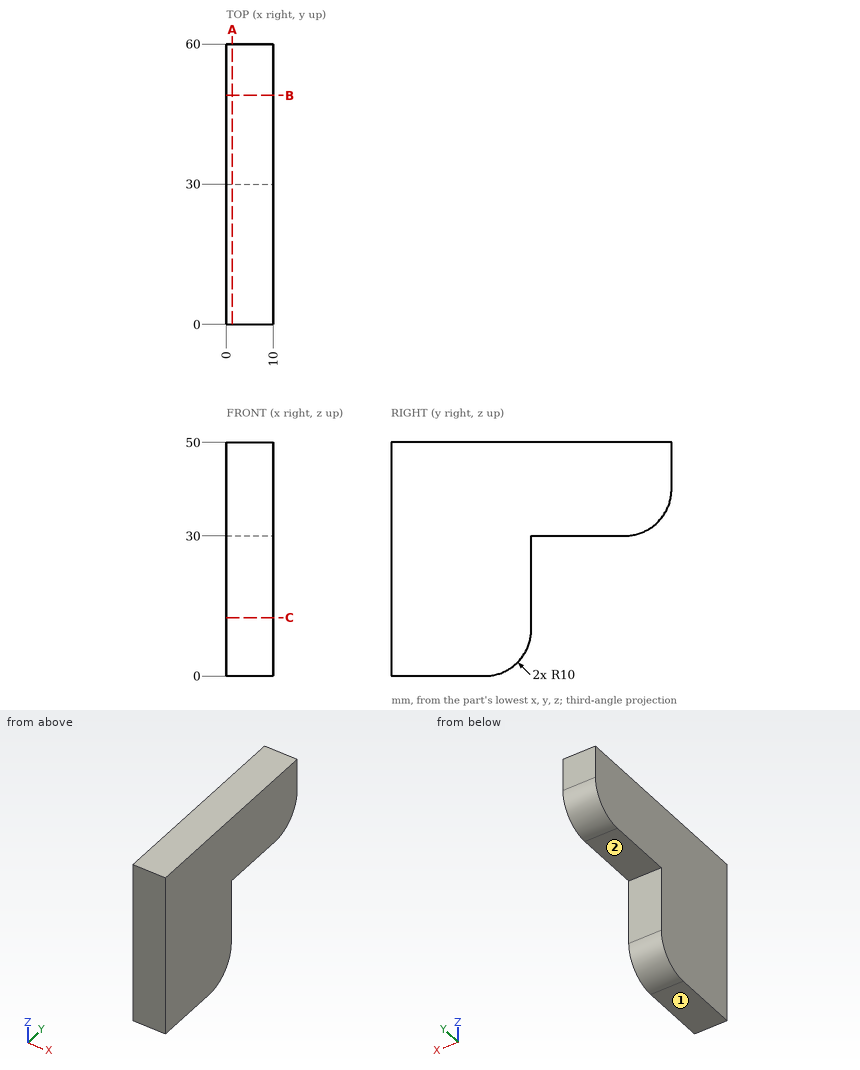
The figure shows three views and two pictorial views of one solid part (mm, origin at its lowest corner). Answer the questions. A direction names the side the tool comes from. Give positions to 0.01 mm unless a question says otherwise; leave off trailing zeros. Loops run counter-clockwise (first coordinate to the right, second up) from the corner with the lowest first, then second, coordinate; pieces in that order, holes last. Notation, with made-up numbers: (50.5, 26) -> (103.5, 26) arc R17 ccw to (103.5, 39) -> close; hole circle Ø9 at (-2.75, 39). An arc over 180 degrees is marked (long way). Put each result on its own line as item: value. Start each with the question number.
Item 1: Which of the six approach directions +Z, -Z, +X, -X, +Y, -Y give full straight-line access (tool end or side, diameter ignored) to the marked faces 1 and 2?
Item 2: Find the intervals of material crossed by L1, parallel to Y at x = 6, z = 18.5; L2, parallel to Z at x = 3, y = 42; L3, parallel to Y at x = 3.5, z = 3, in increasing order. Write a range as [from, to].
Item 3: The part is cut by section C-C (z = 12.5). Give the vertices of the cut face in (x, y).
Item 4: The part is cut by section A-A (x = 1.25). Give the vertices of the cut face in (y, z).
Item 5: Each of these flat-tipped pins is pushed along its axis until it touches: P1, Ø5, axis at x = 3.5, z = 18.5, coming from the +Y side; P2, Ø6, axis at y = 54, z = 39, coming from the -X side; P3, Ø3, axis at x = 3.5, y = 44.5, coming from the -Z side; P4, Ø4, axis at y = 33.5, z = 27, coming from the +X side. Where does it stop, or does it pass through?
Item 6: The part is cut by section B-B (y = 49). Give the vertices of the cut face in (x, z).
Answers below:
1. face 1: -Z, +X, -X, +Y, -Y
1. face 2: -Z, +X, -X, +Y
2. L1: [0, 30]
2. L2: [30, 50]
2. L3: [0, 27.14]
3. outline: (0, 0) -> (10, 0) -> (10, 30) -> (0, 30) -> close
4. outline: (0, 0) -> (20, 0) arc R10 ccw to (30, 10) -> (30, 30) -> (50, 30) arc R10 ccw to (60, 40) -> (60, 50) -> (0, 50) -> close
5. P1: y = 30
5. P2: x = 0
5. P3: z = 30
5. P4: through
6. outline: (0, 30) -> (10, 30) -> (10, 50) -> (0, 50) -> close
